Geometry: final body of the model. Coordinates: model frame, mm. A direction names the side the tool comes from. Round coordinates to 2 decimals unless told otherwise and drop trailing zeros. Write each loop counter-clockwise with the first axis right and the second up, starting at its lowest first coordinate (ties: lowest second). Pieces come first, ordered by that corner, then holes. Notation, with made-up numbers: M 51.5,-33 L 95.5,-33 A18 ccw 95.5,-3 Z; hole C 28.5,71.5 d10. An arc over 180 degrees is marked long. Use one line per item in the form item = value. Start each with the question number.
Item 1: Section query A-A (x = 0). Return loops of the section in (y, z), and give its area (3 significant figures).
Item 2: Ray query, probe 1 along X at (y, z) = (0.2, 0); probe 2 along Y at (x, z) = (16.2, 0); probe 3 along Y at (x, z) = (14, -1.5). Return the intervals inside material, ascending.
Item 3: Section query C-C (y = 4.25). Return loops of the section in (x, z), and give its area (3 significant figures).
Item 4: Section query B-B (z = -1.5). State how many separate pieces and enclosed holes the cut face has, and give its area (3 significant figures).
Item 5: Pin query (flat end, axial travel): pin 1 Ø16 at (x, z) = (0, 0) entering from +Y; pin 2 Ø1.5 at (x, y) = (-6.5, 2.5) entering from +Z; pin 3 Ø2 at (x, y) = (-11, 1) entering from -Z; pin 4 Ø3 at (y, z) = (4.5, -12.5) entering from +X. Return the tip coordinate at first contact, or that it passes through.
Item 6: Reachability of faces 1 (the cylindrical face through (16.52, 0.73, 1.05)), 2 (the cylindrical face through (-13.18, 0.16, -2.93)) from +Z, -Z, +X, -X, +Y, -Y: full face, straight path, thin tool, end or side. Return the list, or none.
Item 7: Pull-direction query (Z, two-part tool) for faces 3 (the cylindrical face through (-17.816, 2.958, -3.956)), 4 (the flat face through (-12, 0, -7)), 5 (the cylindrical face through (-13.18, 5.83, -2.93)); classes: pulls with the +Z half, pulls with the -Z half, needs draft (parallel to the pull), parting line crosses it, or undercut.
from build123d import *

# Parameters (mm, degrees)
SKETCH1_R                 = 18.25
SKETCH1_R_2               = 13.5
BOSS_EXTRUDE1_DEPTH       = 6
SKETCH3_R                 = 2.85
SKETCH4_R                 = 2.5
CUT_EXTRUDE1_DEPTH        = 27.497641404
CUT_EXTRUDE1_DEPTH_BACK   = 10
CUT_EXTRUDE2_REACH        = 28.998
CUT_EXTRUDE2_START_RADIUS = 18.25
CUT_EXTRUDE2_END_RADIUS   = 18.25
SKETCH6_W                 = 1.240344628
SKETCH6_H                 = 0.651674146


with BuildPart() as part:
    # Sketch1 → Boss-Extrude1 (new body)
    with BuildSketch(Plane(origin=(0, 0, 0), x_dir=(1, 0, 0), z_dir=(0, 1, 0))):
        with Locations(Location((0, 0, 0), (0, 0, 270))):
            Circle(SKETCH1_R)
        with Locations(Location((0, 0, 0), (0, 0, 270))):
            Circle(SKETCH1_R_2, mode=Mode.SUBTRACT)
    extrude(amount=BOSS_EXTRUDE1_DEPTH)

    # Sketch3 → Cut-Revolve1 (revolve, cut)
    with BuildSketch(Plane.XY, mode=Mode.PRIVATE) as cut_revolve1_sk:
        with Locations((-12.5, 3)):
            Circle(SKETCH3_R)
    revolve(cut_revolve1_sk.sketch.rotate(Axis((0, 0, 0), (0, 1, 0)), 270), axis=Axis((0, 0, 0), (0, 1, 0)), mode=Mode.SUBTRACT)

    # Sketch4 → Cut-Extrude1 (cut, two sides)
    with BuildSketch(Plane(origin=(0, 0, 0), x_dir=(0, 0, -1), z_dir=(1, 0, 0))) as cut_extrude1_sk:
        with Locations(Location((0, 3, 0), (0, 0, 267.756136347))):
            Circle(SKETCH4_R)
    extrude(amount=CUT_EXTRUDE1_DEPTH, mode=Mode.SUBTRACT)
    extrude(cut_extrude1_sk.sketch, amount=-CUT_EXTRUDE1_DEPTH_BACK, mode=Mode.SUBTRACT)

    # Cut-Extrude2: from a cylinder face, 28.998 long prism both ways, kept between that surface and its translate by the depth
    cut_extrude2_start = Plane(origin=(0, 3, 0), z_dir=(0, -1, 0)) * Cylinder(CUT_EXTRUDE2_START_RADIUS, 95.496, mode=Mode.PRIVATE)
    cut_extrude2_end = Plane(origin=(-0.5, 3, 0), z_dir=(0, -1, 0)) * Cylinder(CUT_EXTRUDE2_END_RADIUS, 95.496, mode=Mode.PRIVATE)
    # Sketch6 → Cut-Extrude2 (cut, from a surface)
    with BuildSketch(Plane(origin=(0, 0, 0), x_dir=(0, 0, -1), z_dir=(1, 0, 0)), mode=Mode.PRIVATE) as cut_extrude2_sk1:
        with Locations((3.176747556, 3)):
            Rectangle(SKETCH6_W, SKETCH6_H)
    cut_extrude2_tool1 = extrude(cut_extrude2_sk1.sketch, amount=CUT_EXTRUDE2_REACH, both=True, mode=Mode.PRIVATE)
    add(((cut_extrude2_tool1 & cut_extrude2_start) - cut_extrude2_end).solids().sort_by_distance((17.710349, 3, -3.176748))[0], mode=Mode.SUBTRACT)


solid = part.part
Working result:
q1.outline = M 0,-18.25 L 6,-18.25 L 6,-13.5 L 5.67,-13.5 A2.85 cw 0.33,-13.5 L 0,-13.5 Z; M 0,13.5 L 0.33,13.5 A2.85 cw 5.67,13.5 L 6,13.5 L 6,18.25 L 0,18.25 Z
q1.area = 42.6 mm²
q2.probe_1 = -18.25 to -13.5, 13.5 to 18.25
q2.probe_2 = 0 to 0.5, 5.5 to 6
q2.probe_3 = 0 to 0.63, 5.37 to 6
q3.outline = M 14.9,-2.17 A15.06 cw long 14.9,2.17 L 18.12,2.17 A18.25 ccw long 18.12,-2.17 Z
q3.area = 320 mm²
q4.separate_pieces = 3
q4.enclosed_holes = 0
q4.area = 30.2 mm²
q5.pin_1 = through
q5.pin_2 = 17.32
q5.pin_3 = -15.27
q5.pin_4 = 14.56
q6.face_1 = +X
q6.face_2 = +Y, -Y
q7.face_3 = parting line crosses it
q7.face_4 = needs draft
q7.face_5 = undercut
